```python
from build123d import *

# Parameters (mm, degrees)
BOSS_EXTRUDE1_DEPTH     = 15
CUT_EXTRUDE1_START      = -7
CUT_EXTRUDE1_DEPTH      = 6.05
CUT_EXTRUDE2_DEPTH      = 29.057975693
CUT_EXTRUDE2_DEPTH_BACK = 29.057975693
CUT_EXTRUDE3_DEPTH      = 29.057975693
CUT_EXTRUDE3_DEPTH_BACK = 29.057975693


with BuildPart() as part:
    # Sketch1 → Boss-Extrude1 (new body)
    with BuildSketch(Plane.XY):
        Polygon((0, 17.5), (0, 0), (17.5, 0), (17.5, 3), (15.5, 3), (3, 15.5), (3, 17.5), align=None)
    extrude(amount=-BOSS_EXTRUDE1_DEPTH)

    # Sketch4 → Cut-Extrude1 (cut, symmetric)
    with BuildSketch(Plane.XY.offset(CUT_EXTRUDE1_START)):
        Polygon((1.5, 17.5), (1.5, 1.5), (17.5, 1.5), (17.5, 3), (3, 17.5), align=None)
    extrude(amount=CUT_EXTRUDE1_DEPTH, both=True, mode=Mode.SUBTRACT)

    # Sketch5 → Cut-Extrude2 (cut, two sides: drawn at the far end of the back side and taken through both)
    with BuildSketch(Plane(origin=(0, 1.5, 0), x_dir=(1, 0, 0), z_dir=(0, 1, 0)).offset(-CUT_EXTRUDE2_DEPTH_BACK)):
        with BuildLine():
            Line((7.5, 8.75), (11.5, 8.75))
            ThreePointArc((11.5, 8.75), (13.25, 7), (11.5, 5.25))
            Line((11.5, 5.25), (7.5, 5.25))
            ThreePointArc((7.5, 5.25), (5.75, 7), (7.5, 8.75))
        make_face()
    extrude(amount=CUT_EXTRUDE2_DEPTH + CUT_EXTRUDE2_DEPTH_BACK, mode=Mode.SUBTRACT)

    # Sketch6 → Cut-Extrude3 (cut, two sides: drawn at the far end of the back side and taken through both)
    with BuildSketch(Plane(origin=(1.5, 0, 0), x_dir=(0, 0, -1), z_dir=(1, 0, 0)).offset(-CUT_EXTRUDE3_DEPTH_BACK)):
        with BuildLine():
            Line((5.25, 7.5), (5.25, 11.5))
            ThreePointArc((5.25, 11.5), (7, 13.25), (8.75, 11.5))
            Line((8.75, 11.5), (8.75, 7.5))
            ThreePointArc((8.75, 7.5), (7, 5.75), (5.25, 7.5))
        make_face()
    extrude(amount=CUT_EXTRUDE3_DEPTH + CUT_EXTRUDE3_DEPTH_BACK, mode=Mode.SUBTRACT)


solid = part.part
```
The model under review builds one solid part; all positions refer to its coordinate system, in mm. A direction names the side the tool comes from. Round coordinates to 2 decimals unless told otherwise and drop trailing zeros. Loops run counter-clockwise (first coordinate to the right, second up) from the corner with the lowest first, then second, coordinate; pieces in that order, holes last. Notation, with made-up numbers: (47, -20) - (89, -20) arc R23 cw to (89, 8) - close; hole circle Ø6 at (2.25, 78). An arc over 180 degrees is marked (long way). Write each question's results on one line, items separated by ' | '. Start each with the question number.
Q1. Wall thickness on line 1 along Z through (x, y) = (6, 9.75); line 2 along Z through (x, y) = (0.75, 9); line 3 along X through (y, z) = (13, -3.25): over which ranges is each line inside the solid? List them lowest first. Write a range as [from, to].
Q2. Draft analysis for pull direction Z (two halves, no side actions). For faces 1 (the flat face through (1, 9, -5.25)), 2 (the flat face through (7, 7, -15)), 3 (the flat face through (17.5, 1, -7)), state which applies: pulls with the +Z half, pulls with the -Z half, needs draft (parallel to the pull), parting line crosses it, or undercut.
Q3. Take a section at A-A on z = -7. Give the boundary of the cut face in (x, y), plus the area to 4 significant figures.
Q4. Insertion check: P1, Ø4, axis at x = 14, z = -2.5, coming from the +Y side; P2, Ø4, axis at x = 7.5, y = 14, coming from the +Z side; P3, Ø1, axis at y = 17, z = -14.5, coming from the +X side; P4, Ø1.6, axis at x = 16.5, z = -14, coming from the +Y side. Each pin has a flat end and moves straight along its axis. Give the tip position at first contact, or say it passes through.
Q5. Take a section at B-B on y = 10.25. Give the boundary of the cut face in (x, z).
Q6. Tool access review of faces 4 (the flat face through (9, 1.5, -10)), 5 (the flat face through (1, 10, -8.75)), 6 (the flat face through (9, 1, -8.75)): name each direction out of +Z, -Z, +X, -X, +Y, -Y from which nothing blocks a thin tool from reaching the whole face with its end or side.
Q7. Take a section at D-D on z = -4. Give the boundary of the cut face in (x, y), plus the area to 4 significant figures.
Q8. Take a section at C-C on x = 2.75. Give the boundary of the cut face in (y, z), plus the area to 3 significant figures.
Data:
1) line 1: z = [-15, -13.05], [-0.95, 0] | line 2: z = [-15, -8.75], [-5.25, 0] | line 3: x = [0, 1.5]
2) face 1: undercut | face 2: pulls with the -Z half | face 3: needs draft
3) outline: (0, 0) - (5.75, 0) - (5.75, 1.5) - (1.5, 1.5) - (1.5, 5.75) - (0, 5.75) - close; (0, 13.25) - (1.5, 13.25) - (1.5, 17.5) - (0, 17.5) - close; (13.25, 0) - (17.5, 0) - (17.5, 1.5) - (13.25, 1.5) - close | area: 27.75 mm²
4) P1: stops at y = 5.76 | P2: passes through | P3: stops at x = 3 | P4: stops at y = 3
5) outline: (0, -15) - (8.25, -15) - (8.25, -13.05) - (1.5, -13.05) - (1.5, -8.75) - (0, -8.75) - close; (0, -5.25) - (1.5, -5.25) - (1.5, -0.95) - (8.25, -0.95) - (8.25, 0) - (0, 0) - close
6) face 4: +X, +Y | face 5: +X, -X | face 6: +Y, -Y
7) outline: (0, 0) - (17.5, 0) - (17.5, 1.5) - (1.5, 1.5) - (1.5, 17.5) - (0, 17.5) - close | area: 50.25 mm²
8) outline: (0, -15) - (17.5, -15) - (17.5, -13.05) - (1.5, -13.05) - (1.5, -0.95) - (17.5, -0.95) - (17.5, 0) - (0, 0) - close | area: 68.9 mm²
